Drawing for the job (mm, zero at the part's lowest x, y, z). Give positions to 0.01 mm unless a question says otherwise; leave off trailing zeros. Loops run counter-clockwise (first coordinate to the right, second up) from the corner with the lowest first, then second, coordinate; pieces in that order, holes last.
1) Band-saw the part on D-D on y = 2.2. State how many separate pieces and enclosed holes the cut face has, then the cut area to 3 significant figures.
2) Band-saw the part on C-C on x = 8.5. List the corners of the cut face in (y, z), then the cut area to 3 significant figures.
3) Flat gauge pins, fed straight in: P1, Ø3, axis at y = 3.5, z = 36, coming from the +X side; P2, Ø1.5, axis at x = 9, y = 3.5, coming from the -Z side; P3, Ø3, axis at x = 17.5, y = 3, coming from the +Z side; P4, Ø2.5, axis at x = 91.5, z = 50, coming from the +Y side. Where does each tip first touch, or does it go through?
4) Band-saw the part on A-A on x = 50. List the corners of the cut face in (y, z), then the cut area to 3 significant figures.
5) Wall check: line 1 (Z direction, x = 91.5, y = 3.5); line 2 (Z direction, x = 80, y = 1.7); line 3 (X direction, y = 3.15, z = 59.5). Give the ranges that are in metal, low to high.
6) Band-saw the part on B-B on z = 60. List the corners of the cut face in (x, y).
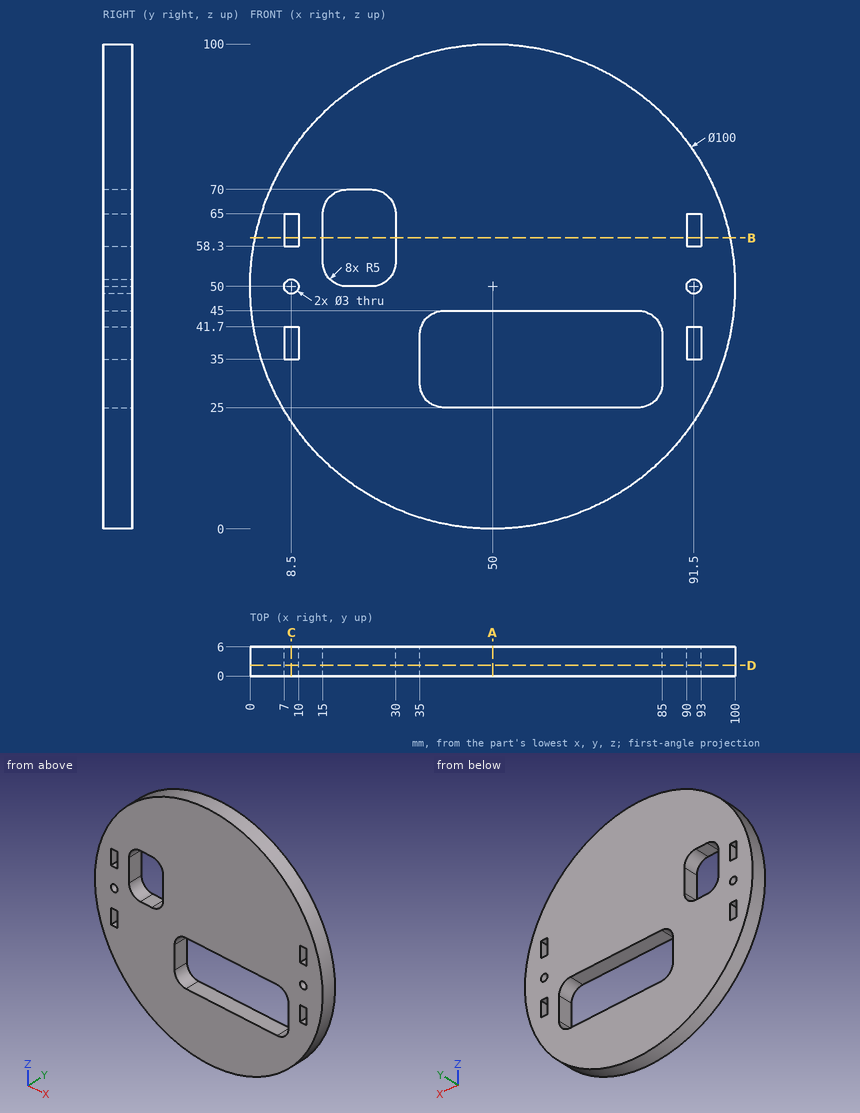
Findings below:
1. separate pieces: 1
1. enclosed holes: 8
1. area: 6,500 mm2
2. outline: (0, 22.11) - (6, 22.11) - (6, 35) - (0, 35) - close; (0, 41.7) - (6, 41.7) - (6, 48.5) - (0, 48.5) - close; (0, 51.5) - (6, 51.5) - (6, 58.3) - (0, 58.3) - close; (0, 65) - (6, 65) - (6, 77.89) - (0, 77.89) - close
2. area: 236 mm2
3. P1: stops at x = 98.41
3. P2: stops at z = 20.34
3. P3: stops at z = 89.23
3. P4: passes through
4. outline: (0, 0) - (6, 0) - (6, 25) - (0, 25) - close; (0, 45) - (6, 45) - (6, 100) - (0, 100) - close
4. area: 480 mm2
5. line 1: z = 22.11 to 35, 41.7 to 48.5, 51.5 to 58.3, 65 to 77.89
5. line 2: z = 10 to 25, 45 to 90
5. line 3: x = 0.91 to 7, 10 to 15, 30 to 90, 93 to 99.09
6. outline: (1.01, 0) - (7, 0) - (7, 6) - (1.01, 6) - close; (10, 0) - (15, 0) - (15, 6) - (10, 6) - close; (30, 0) - (90, 0) - (90, 6) - (30, 6) - close; (93, 0) - (98.99, 0) - (98.99, 6) - (93, 6) - close
